from build123d import *

# Parameters (mm, degrees)
SKETCH1_W               = 63
SKETCH1_H               = 60
BOSS_EXTRUDE1_DEPTH     = 30
SKETCH2_W               = 60
SKETCH2_H               = 57
CUT_EXTRUDE1_DEPTH      = 44
FILLET5_R               = 1
FILLET6_R               = 1
SKETCH4_W               = 11.2479448
SKETCH4_H               = 1.120832932
BOSS_EXTRUDE2_DEPTH     = 4
SKETCH7_W               = 11.602367515
SKETCH7_H               = 0.946433532
BOSS_EXTRUDE3_DEPTH     = 4
SKETCH13_W              = 60
SKETCH13_H              = 1.5
BOSS_EXTRUDE4_DEPTH     = 52
SKETCH8_R               = 2.75
CUT_EXTRUDE2_DEPTH      = 15
CUT_EXTRUDE2_DEPTH_BACK = 20
SKETCH18_W              = 10
SKETCH18_H              = 5
CUT_EXTRUDE4_DEPTH      = 15


with BuildPart() as part:
    # Sketch1 → Boss-Extrude1 (new body)
    with BuildSketch(Plane(origin=(0, 0, 0), x_dir=(1, 0, 0), z_dir=(0, 1, 0))):
        with Locations((8.284946237, -2.70609319)):
            Rectangle(SKETCH1_W, SKETCH1_H)
    extrude(amount=BOSS_EXTRUDE1_DEPTH)

    # Sketch2 → Cut-Extrude1 (cut)
    with BuildSketch(Plane(origin=(0, 0, 0), x_dir=(1, 0, 0), z_dir=(0, 1, 0))):
        with Locations((8.284946237, -2.70609319)):
            Rectangle(SKETCH2_W, SKETCH2_H)
    extrude(amount=CUT_EXTRUDE1_DEPTH, mode=Mode.SUBTRACT)

    # Fillet5
    fillet5_edges = [part.edges().sort_by_distance(p)[0] for p in [
        (39.784946237, 15, -27.29390681),
    ]]
    fillet(fillet5_edges, radius=FILLET5_R)

    # Fillet6
    fillet6_edges = [part.edges().sort_by_distance(p)[0] for p in [
        (-23.215053763, 15, -27.29390681),
        (39.784946237, 15, 32.70609319),
        (-23.215053763, 15, 32.70609319),
    ]]
    fillet(fillet6_edges, radius=FILLET6_R)

    # Sketch4 → Boss-Extrude2 (add)
    with BuildSketch(Plane(origin=(-21.715053763, 0, 0), x_dir=(0, 0, -1), z_dir=(1, 0, 0))):
        with Locations((-6.456507936, 29.439583534)):
            Rectangle(SKETCH4_W, SKETCH4_H)
    extrude(amount=BOSS_EXTRUDE2_DEPTH)

    # Sketch7 → Boss-Extrude3 (add)
    with BuildSketch(Plane.ZY.offset(-38.284946237)):
        with Locations((6.279296579, 29.526783234)):
            Rectangle(SKETCH7_W, SKETCH7_H)
    extrude(amount=BOSS_EXTRUDE3_DEPTH)

    # Sketch13 → Boss-Extrude4 (add)
    with BuildSketch(Plane.XY.offset(-25.79390681)):
        with Locations((8.284946237, 0.75)):
            Rectangle(SKETCH13_W, SKETCH13_H)
    extrude(amount=BOSS_EXTRUDE4_DEPTH)

    # Sketch8 → Cut-Extrude2 (cut, two sides)
    with BuildSketch(Plane.XY.offset(32.70609319)) as cut_extrude2_sk:
        with Locations((-2.391644106, 23.745075348)):
            Circle(SKETCH8_R)
    extrude(amount=CUT_EXTRUDE2_DEPTH, mode=Mode.SUBTRACT)
    extrude(cut_extrude2_sk.sketch, amount=-CUT_EXTRUDE2_DEPTH_BACK, mode=Mode.SUBTRACT)

    # Sketch18 → Cut-Extrude4 (cut)
    with BuildSketch(Plane(origin=(39.784946237, 0, 0), x_dir=(0, 0, -1), z_dir=(1, 0, 0))):
        with Locations((9.363418395, 14.577492713)):
            Rectangle(SKETCH18_W, SKETCH18_H)
    extrude(amount=-CUT_EXTRUDE4_DEPTH, mode=Mode.SUBTRACT)


solid = part.part
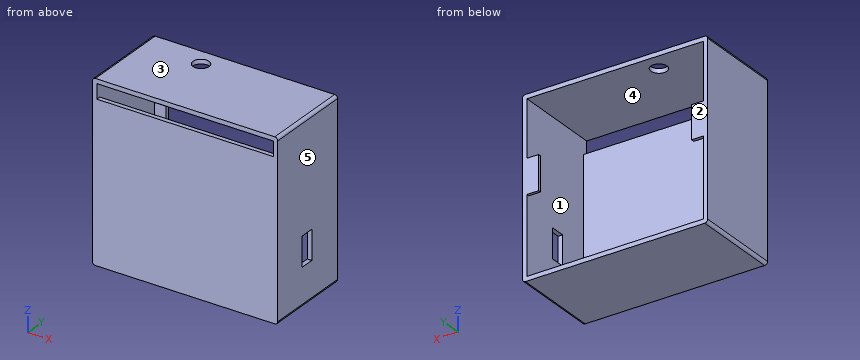
Geometry: final body of the model. Coordinates: model frame, mm. Face numbers are marked on the shaded views. A direction names the side the tool comes from. Coordinates: 2 decimals unless noted, no trailing zeros. Order: outer loops, then holes, each group sorted by start corner. A loop starts at its lowest first (then second) coordinate and runs counter-clockwise, first axis right, second up. Notation, with made-up numbers: M 81.5,-7 L 135.5,-7 A18 ccw 135.5,6 Z; hole C 84,-28 d9. An arc over 180 degrees is marked long. One line per question, with ' | ' between items. Start each with the question number.
Item 1: Ray query, probe 1 along Z at (x, y) = (0.5, 8.25); probe 2 along X at (y, z) = (25, -4); probe 3 along Y at (x, z) = (14, 17). Return the intervals inside material, ascending. Write a range as [from, to].
Item 2: Cut plane D-D, the plane z = -22. Return the cut outline in (x, y), then the cut area to 3 significant figures.
Item 3: Set-up query: the marked faces 4 and 5. Return all of +Z, -Z, +X, -X, +Y, -Y with unobstructed straight access to the full face (end or side cutting, diameter ignored); none if empty.
Item 4: Cut plane C-C, the plane y = 16. Return the cut outline in (x, z), then the cut area to 3 significant figures.
Item 5: Cut plane B-B, the plane y = 8. Return the cut outline in (x, z).
Item 6: Cut plane A-A, the plane x = -16. Return the cut outline in (y, z).
Item 7: Pin query (flat end, axial travel): pin 1 Ø4 at (x, z) = (29.5, -11) entering from -Y. Return the tip coordinate at first contact, or that it passes through.
Item 8: Draft query along Y for the marked faces 1, 2 and 3. Return one class per face: released by +Y, released by -Y, zero draft, split by the parting line, or undercut.
A:
1) probe 1: z = [-27.29, -25.79], [31.21, 32.71] | probe 2: x = [-23.22, -21.72], [38.28, 39.78] | probe 3: y = [0, 1.5]
2) outline: M -23.22,0 L 39.78,0 L 39.78,30 L 38.28,30 L 38.28,1.5 L -21.72,1.5 L -21.72,30 L -23.22,30 Z | area: 180 mm2
3) face 4: +Y, -Y | face 5: +Z, -Z, +X, +Y, -Y
4) outline: M -23.22,-26.29 A1 ccw -22.22,-27.29 L 38.78,-27.29 A1 ccw 39.78,-26.29 L 39.78,-14.36 L 38.28,-14.36 L 38.28,-25.79 L -21.72,-25.79 L -21.72,31.21 L 38.28,31.21 L 38.28,-4.36 L 39.78,-4.36 L 39.78,31.71 A1 ccw 38.78,32.71 L -22.22,32.71 A1 ccw -23.22,31.71 Z | area: 344 mm2
5) outline: M -23.22,-26.29 A1 ccw -22.22,-27.29 L 38.78,-27.29 A1 ccw 39.78,-26.29 L 39.78,31.71 A1 ccw 38.78,32.71 L -22.22,32.71 A1 ccw -23.22,31.71 Z; hole M -21.72,-25.79 L 38.28,-25.79 L 38.28,31.21 L -21.72,31.21 Z
6) outline: M 0,-27.29 L 30,-27.29 L 30,-25.79 L 1.5,-25.79 L 1.5,26.21 L 0,26.21 Z; M 0,31.21 L 30,31.21 L 30,32.71 L 0,32.71 Z
7) pin 1: stops at y = 0
8) face 1: undercut | face 2: released by +Y | face 3: zero draft
